Print and shaded views of the part. All mm, measured from the part's lowest x, y and z. A direction names the side the tool comes from. Coordinates: 2 decimals unless noted, no trailing zeros. Loops run counter-clockwise (first coordinate to the right, second up) from the corner with the lowest first, then second, coordinate; pieces in that order, holes last.
1) Saw through at C-C, the plane x = 4. Write the cut outline in (y, z), and give its area (3 significant figures).
2) Pin check, flat tips, straight feed: pin 1 Ø3 at (y, z) = (4.5, 6.5) entering from +X; pin 2 Ø2.5 at (x, y) = (20.93, 4) entering from +Z. Stop position of each tip, or through.
3) Saw through at B-B, the plane y = 4. Write the cut outline in (x, z), and give its area (3 significant figures).
4) Saw through at D-D, the plane y = 7.75. Write the cut outline in (x, z).
5) Which spindle directions (+Z, -Z, +X, -X, +Y, -Y) get a long thin tool onto all of the face, cutting with end or side? Do the marked faces 4 and 5. Say none if no direction does.
6) Wall check: line 1 along X through (y, z) = (5, 3.5) (1 decimal); line 2 along X through (y, z) = (3.25, 7.25) (1 decimal); line 3 along Y through (x, z) = (4, 2.25). Give the ranges that are in metal, low to high.
7) Saw through at A-A, the plane z = 5.5. Write the cut outline in (x, y).
8) Two-plate mould, pull along X, no slides. Class the marked faces 1, 2 and 3: +X half, -X half, draft (parallel to the pull), parting line (faces both ways), or undercut.
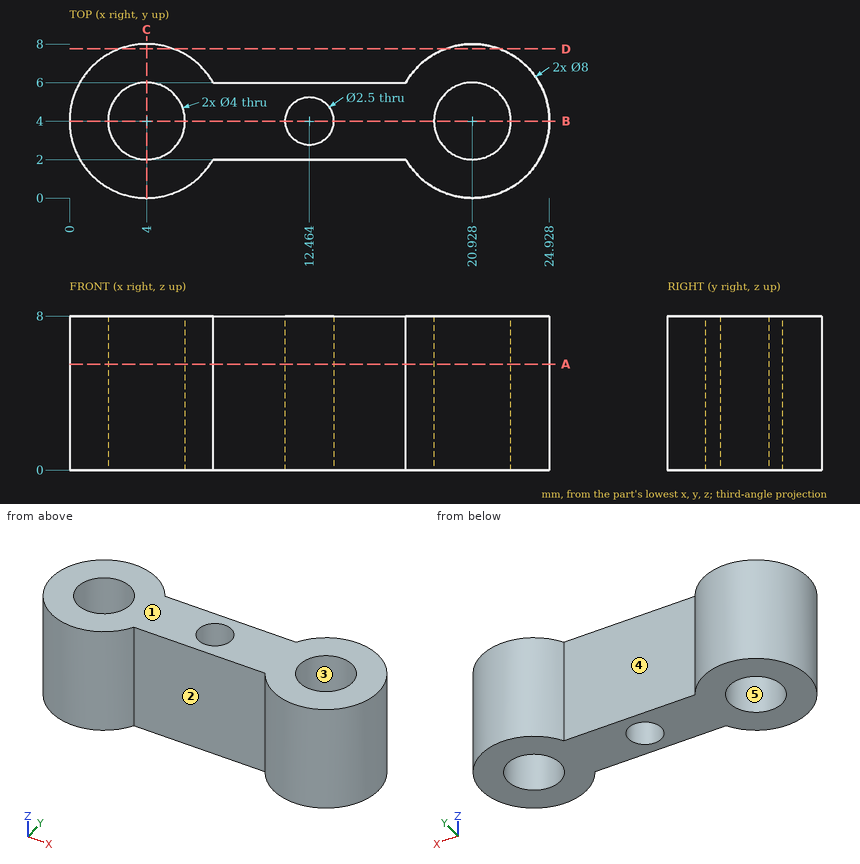
Data:
1. outline: (0, 0) - (2, 0) - (2, 8) - (0, 8) - close; (6, 0) - (8, 0) - (8, 8) - (6, 8) - close
1. area: 32.0 mm2
2. pin 1: stops at x = 24.93
2. pin 2: passes through
3. outline: (0, 0) - (2, 0) - (2, 8) - (0, 8) - close; (6, 0) - (11.21, 0) - (11.21, 8) - (6, 8) - close; (13.71, 0) - (18.93, 0) - (18.93, 8) - (13.71, 8) - close; (22.93, 0) - (24.93, 0) - (24.93, 8) - (22.93, 8) - close
3. area: 115 mm2
4. outline: (2.61, 0) - (5.39, 0) - (5.39, 8) - (2.61, 8) - close; (19.54, 0) - (22.32, 0) - (22.32, 8) - (19.54, 8) - close
5. face 4: +Z, -Z, +Y
5. face 5: +Z, -Z
6. line 1: x = 0.1 to 2.3, 5.7 to 11.7, 13.2 to 19.2, 22.7 to 24.8
6. line 2: x = 0.1 to 2.1, 5.9 to 11.5, 13.5 to 19.1, 22.8 to 24.9
6. line 3: y = 0 to 2, 6 to 8
7. outline: (7.46, 2) - (17.46, 2) arc R4 ccw (long way) to (17.46, 6) - (7.46, 6) arc R4 ccw (long way) to start; hole circle Ø4 at (4, 4); hole circle Ø2.5 at (12.46, 4); hole circle Ø4 at (20.93, 4)
8. face 1: draft
8. face 2: undercut
8. face 3: undercut
